Geometry check sheet. Reference: the model listing, model coordinates, mm. A direction names the side the tool comes from. Coordinates: 2 decimals unless noted, no trailing zeros. Write each loop counter-clockwise with the first axis right and the second up, starting at its lowest first coordinate (ties: lowest second). Pieces come first, ordered by that corner, then holes. Notation, with made-up numbers: (74, 4.5) -> (107, 4.5) arc R19 cw to (107, 20.5) -> close; hole circle Ø7 at (81, -0.75). An arc over 180 degrees is marked (long way). Put each result on its own line as item: value. Start each with the question number.
from build123d import *

# Parameters (mm, degrees)
EXTRUDE_1_DEPTH     = 30.144123077
SKETCH_2_W          = 100
SKETCH_2_H          = 100
EXTRUDE_1_2_DEPTH   = 30.144123077
SKETCH_3_R          = 7.5
CUT_EXTRUDE_1_DEPTH = 10
CUT_EXTRUDE_3_DEPTH = 31.144123077


with BuildPart() as part:
    # Sketch 2 → Extrude 1 (new body)
    with BuildSketch(Plane(origin=(0, 0, 0), x_dir=(1, 0, 0), z_dir=(0, 1, 0))):
        Polygon((80, 50), (80, -50), (180, -50), align=None)
    extrude(amount=EXTRUDE_1_DEPTH)


with BuildPart() as body_2:
    # Sketch 2 → Extrude 1 2 (new body)
    with BuildSketch(Plane(origin=(0, 0, 0), x_dir=(1, 0, 0), z_dir=(0, 1, 0))):
        Rectangle(SKETCH_2_W, SKETCH_2_H)
    extrude(amount=EXTRUDE_1_2_DEPTH)

    # Sketch 3 → Cut-Extrude 1 (cut)
    with BuildSketch(Plane(origin=(0, 30.144123077, 0), x_dir=(1, 0, 0), z_dir=(0, 1, 0))):
        Circle(SKETCH_3_R)
        with BuildLine():
            Line((-25, -22.5), (25, -22.5))
            ThreePointArc((25, -22.5), (32.5, -30), (25, -37.5))
            Line((25, -37.5), (-25, -37.5))
            ThreePointArc((-25, -37.5), (-32.5, -30), (-25, -22.5))
        make_face()
    extrude(amount=-CUT_EXTRUDE_1_DEPTH, mode=Mode.SUBTRACT)


with BuildPart() as body_3:
    # Mirror 2: mirrored copy
    add(part.part.mirror(Plane(origin=(0, 0, 0), x_dir=(0, 0, 1), z_dir=(1, 0, 0))))


with BuildPart() as cut_extrude_3_tool:
    # Sketch 6 → Cut-Extrude 3 (new body, through all)
    with BuildSketch(Plane(origin=(0, 30.144123077, 0), x_dir=(1, 0, 0), z_dir=(0, 1, 0))):
        Polygon((80, 50), (80, -50), (180, -50), align=None)
        Polygon((-80, 50), (-180, -50), (-80, -50), align=None)
    extrude(amount=-CUT_EXTRUDE_3_DEPTH)


with BuildPart() as part_1:
    add(part.part)

    # Cut-Extrude 3: cut by cut_extrude_3_tool
    add(cut_extrude_3_tool.part, mode=Mode.SUBTRACT)


with BuildPart() as body_3_1:
    add(body_3.part)

    # Cut-Extrude 3: cut by cut_extrude_3_tool
    add(cut_extrude_3_tool.part, mode=Mode.SUBTRACT)


solid = body_2.part
Item 1: Access from +Z, -Z, +X, -X, +Y, -Y to the whole of each face (thin tool, end or side, straight path). Record for faces 1 (the flat face through (-1, 30.144, -12)), 2 (the flat face through (0, 25, 37.5)).
Item 2: Section check B-B, the plane z = 30. Enter the section's corners in (x, y).
Item 3: Section check A-A, the plane y = 23.5. Enter the section's corners in (x, z), and give its area (3 significant figures).
Item 4: Scan lines: line 1 along Z through (x, y) = (0, 28.25); line 2 along X through (y, z) = (22.5, 0); line 3 along Z through (x, y) = (8, 25.5). Record each from-to range of solid material in increasing order. Write a range as [from, to].
Item 5: Section check C-C, the plane x = 9. Enter the section's corners in (y, z), and give its area (3 significant figures).
Item 6: Mould release check, pull along X, two halves, no side actions. Record for faces 3 (the flat face through (50, 15, 1)), 4 (the cylindrical face through (32.5, 25.21, 29.84)), 5 (the flat face through (-1, 15, 50)): released by +X, released by -X, zero draft, split by the parting line, or undercut.
Item 7: Go/stop test with a flat-tipped pin: P1, Ø7.5, axis at x = 14.5, z = 32.5, coming from the +Y side. Record where the tip stops, or that it passes through.
From the geometry:
1. face 1: +Z, -Z, +X, -X, +Y
1. face 2: +Y
2. outline: (-50, 0) -> (50, 0) -> (50, 30.14) -> (32.5, 30.14) -> (32.5, 20.14) -> (-32.5, 20.14) -> (-32.5, 30.14) -> (-50, 30.14) -> close
3. outline: (-50, -50) -> (50, -50) -> (50, 50) -> (-50, 50) -> close; hole (-25, 22.5) -> (25, 22.5) arc R7.5 ccw to (25, 37.5) -> (-25, 37.5) arc R7.5 ccw to start; hole circle Ø15 at (0, 0)
3. area: 8,900 mm²
4. line 1: [-50, -7.5], [7.5, 22.5], [37.5, 50]
4. line 2: [-50, -7.5], [7.5, 50]
4. line 3: [-50, 22.5], [37.5, 50]
5. outline: (0, -50) -> (30.14, -50) -> (30.14, 22.5) -> (20.14, 22.5) -> (20.14, 37.5) -> (30.14, 37.5) -> (30.14, 50) -> (0, 50) -> close
5. area: 2,860 mm²
6. face 3: released by +X
6. face 4: undercut
6. face 5: zero draft
7. P1: y = 20.14
